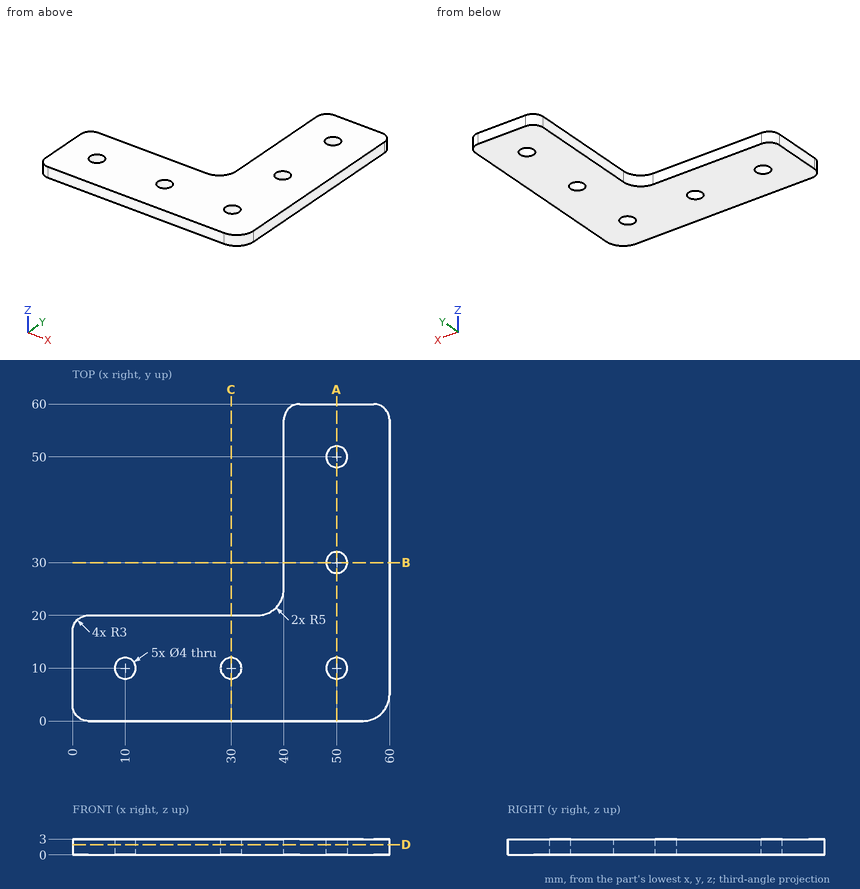
For this review, use the dimensioned drawing (mm, ordinates from the lowest corner) and the shaded views. Round coordinates to 2 decimals unless told otherwise and drop trailing zeros. Order: outer loops, then holes, each group sorted by start corner. A loop starts at its lowest first (then second) coordinate and runs counter-clockwise, first axis right, second up. Notation, with made-up numbers: M 15,-19.75 L 47,-19.75 A12 ccw 47,-4.75 Z; hole C 37,7.5 d3. An arc over 180 degrees is marked long. Write each question's results on one line, items separated by ' | '. Start each with the question number.
1. Add section B-B (y = 30). State the section outline as (x, z) points, then the cut area to 3 significant figures.
2. Clearance check with flat-ended pins moving along their axes: pin 1 Ø6.5 at (x, y) = (10, 10) entering from -Z; pin 2 Ø0.9 at (y, z) = (35, 1.5) entering from -X. State where each tip first meets the part, or that it passes through.
3. Add section A-A (x = 50). State the section outline as (y, z) points.
4. Add section D-D (z = 1.95). State the section outline as (x, y) points, then the cut area to 3 significant figures.
5. Add section C-C (x = 30). State the section outline as (y, z) points.
6. To check wall thickness, follow L1, parallel to Y at x = 50, z = 1.55; L2, parallel to Y at x = 10, z = 0.75; L3, parallel to X at y = 46.5, z = 2.75. State the ranges of each line that lie inside material, in increasing order. Write a range as [from, to].
Output values:
1) outline: M 40,0 L 48,0 L 48,3 L 40,3 Z; M 52,0 L 60,0 L 60,3 L 52,3 Z | area: 48.0 mm^2
2) pin 1: z = 0 | pin 2: x = 40
3) outline: M 0,0 L 8,0 L 8,3 L 0,3 Z; M 12,0 L 28,0 L 28,3 L 12,3 Z; M 32,0 L 48,0 L 48,3 L 32,3 Z; M 52,0 L 60,0 L 60,3 L 52,3 Z
4) outline: M 0,3 A3 ccw 3,0 L 55,0 A5 ccw 60,5 L 60,57 A3 ccw 57,60 L 43,60 A3 ccw 40,57 L 40,25 A5 cw 35,20 L 3,20 A3 ccw 0,17 Z; hole C 10,10 d4; hole C 30,10 d4; hole C 50,10 d4; hole C 50,30 d4; hole C 50,50 d4 | area: 1,930 mm^2
5) outline: M 0,0 L 8,0 L 8,3 L 0,3 Z; M 12,0 L 20,0 L 20,3 L 12,3 Z
6) L1: [0, 8], [12, 28], [32, 48], [52, 60] | L2: [0, 8], [12, 20] | L3: [40, 60]
